Part print with two shaded views. Sizes in mm from the minimum x, y, z corner. Coordinates: 2 decimals unless noted, no trailing zeros. Loops run counter-clockwise (first coordinate to the right, second up) from the corner with the lowest first, then second, coordinate; pieces in that order, holes last. Notation, with made-up numbers: (17, 82) -> (63, 82) arc R30 ccw to (63, 114) -> close; hole circle Ø2 at (87, 61). An arc over 180 degrees is marked (long way). Use one line per item in the form item = value.
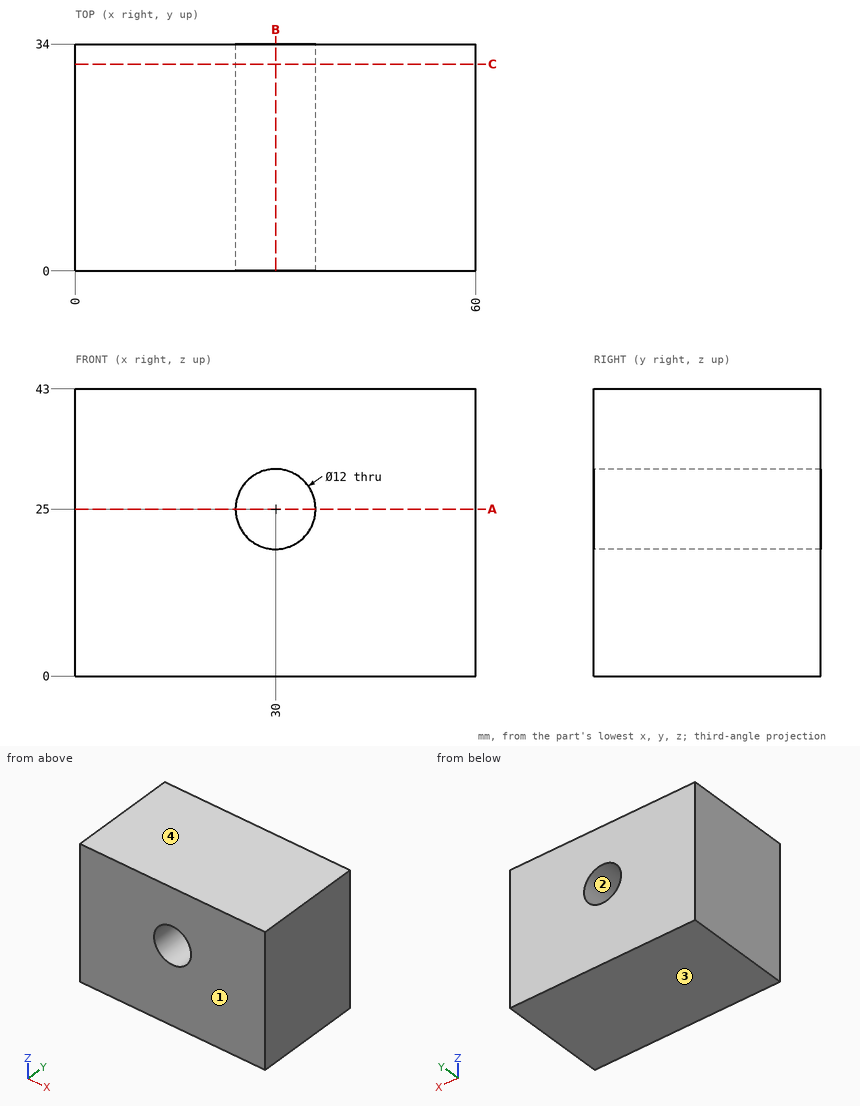
Q1. Band-saw the part on A-A, the plane z = 25. Write the cut outline in (x, y).
Result:
outline = (0, 0) -> (24, 0) -> (24, 34) -> (0, 34) -> close; (36, 0) -> (60, 0) -> (60, 34) -> (36, 34) -> close
Q2. Wall check: line 1 along Z through (x, y) = (30, 10); line 2 along Z through (x, y) = (35.5, 9.5); line 3 along X through (y, z) = (14, 26). Give the ranges that are in metal, low to high.
Result:
line_1 = 0 to 19, 31 to 43
line_2 = 0 to 22.6, 27.4 to 43
line_3 = 0 to 24.08, 35.92 to 60
Q3. Band-saw the part on B-B, the plane x = 30. Write the cut outline in (y, z), and give its area (3 significant figures).
Result:
outline = (0, 0) -> (34, 0) -> (34, 19) -> (0, 19) -> close; (0, 31) -> (34, 31) -> (34, 43) -> (0, 43) -> close
area = 1,050 mm2
Q4. Band-saw the part on C-C, the plane y = 31. Write the cut outline in (x, z).
Result:
outline = (0, 0) -> (60, 0) -> (60, 43) -> (0, 43) -> close; hole circle Ø12 at (30, 25)
Q5. Pin check, flat tip, straight feed: pin 1 Ø1 at (x, z) = (34.5, 25) entering from +Y. Stop position of the tip, or through.
Result:
pin_1 = through
Q6. Mould opens along Z. For the marked faces 1, 2, 3 and 4 say: released by +Z, released by -Z, zero draft, split by the parting line, or undercut.
Result:
face_1 = zero draft
face_2 = undercut
face_3 = released by -Z
face_4 = released by +Z
